Design review of the part built by this model. Coordinates are the model's own, in mm. A direction names the side the tool comes from. Give positions to 0.01 mm unless a question says otherwise; leave off trailing zeros. Loops run counter-clockwise (first coordinate to the right, second up) from the corner with the lowest first, then second, coordinate; pieces in that order, holes last. Notation, with made-up numbers: (83, -35) -> (121, -35) arc R21 ccw to (121, -15) -> close; hole circle Ø4 at (77.5, 30). An arc over 180 degrees is marked (long way). Use a Markdown table: item, result. Add a question column.
1. Add section C-C (z = 5.4). State the section outline as (x, y) points.
2. For faces 1 (the cylindrical face through (-10.46, -6.16, 4.04)), 2 (the flat face through (4.35, 2.465, 2.958)), 3 (the flat face through (7.5, 10, 3)), 4 (the flat face through (-4.556, -11.29, 2.958)), list the 3-axis set-ups (+Z, -Z, +X, -X, +Y, -Y) from which the entire face can be reached by the end or side of a thin tool; tool diameter is ignored.
3. To check wall thickness, follow line 1 (Z direction, x = -2, y = 12); line 2 (X direction, y = -8.25, z = 2.75); line 3 (X direction, y = -4.75, z = 4.1). State the ranges of each line that lie inside material, in increasing order.
4. Draft analysis for pull direction X (two halves, no side actions). For faces 5 (the flat face through (4.556, -11.29, 2.958)), 6 (the flat face through (0, 15, 3)), 7 (the cylindrical face through (9.58, -5.41, 3.32)), 8 (the flat face through (-7.5, 10, 3)), state which applies: pulls with the +X half, pulls with the -X half, needs draft (parallel to the pull), parting line crosses it, or undercut.
5. Add section D-D (z = 3). State the section outline as (x, y) points, and give its area (3 significant figures).
6. Add section A-A (y = 12). State the section outline as (x, z) points.
7. For pin 1 Ø2 at (y, z) = (8.5, 1.5) entering from -X; pin 2 Ø1.3 at (y, z) = (12, 3) entering from +X, all flat-tipped, find the tip position at first contact; note any pin that passes through.
8. Add section B-B (x = -5). State the section outline as (y, z) points.
```python
from build123d import *

# Parameters (mm, degrees)
F0_W     = 15
F0_H     = 15
F1_DEPTH = 6
F2_R     = 1.05
F3_DEPTH = 15
F5_COUNT = 3
F7_DEPTH = 6


with BuildPart() as f1:
    # F0 (on Top) → F1 (new body)
    with BuildSketch(Plane.XY):
        with Locations((0, 7.5)):
            Rectangle(F0_W, F0_H)
    extrude(amount=F1_DEPTH)

    # F2 (on face) → F3 (cut, through all)
    with BuildSketch(Plane(origin=(-7.5, 0, 0), x_dir=(0, -1, 0), z_dir=(-1, 0, 0))):
        with Locations((-12, 3)):
            Circle(F2_R)
    extrude(amount=-F3_DEPTH, mode=Mode.SUBTRACT)

    # F5: F1 ×3 about axis
    f5_axis = Axis((0, 0, -1.369192), (0, 0, -1))


with BuildPart() as f1_1:
    add(f1.part)
    for i in range(1, F5_COUNT):
        add(f1.part.rotate(f5_axis, i * 360 / F5_COUNT))

    # F6 (on Top) → F7 (cut, through all)
    with BuildSketch(Plane.XY):
        Polygon((2.886751, 5), (-2.886751, 5), (-5.773503, 0), (-2.886751, -5), (2.886751, -5), (5.773503, 0), align=None)
    extrude(amount=F7_DEPTH, mode=Mode.SUBTRACT)


solid = f1_1.part
```
Taken from the geometry:
| question | item | result |
|---|---|---|
| 1 | outline | (-16.74, -1) -> (-9.24, -14) -> (0, -8.66) -> (9.24, -14) -> (16.74, -1) -> (7.5, 4.33) -> (7.5, 15) -> (-7.5, 15) -> (-7.5, 4.33) -> close; hole (-5.77, 0) -> (-2.89, -5) -> (2.89, -5) -> (5.77, 0) -> (2.89, 5) -> (-2.89, 5) -> close |
| 2 | face 1 | none |
| 2 | face 2 | +Z, -Z |
| 2 | face 3 | +Z, -Z, +X, +Y |
| 2 | face 4 | +Z, -Z, -Y |
| 3 | line 1 | z = 0 to 1.95, 4.05 to 6 |
| 3 | line 2 | x = -12.56 to -10.27, -7.92 to 7.92, 10.27 to 12.56 |
| 3 | line 3 | x = -14.58 to -3.03, 3.03 to 14.58 |
| 4 | face 5 | undercut |
| 4 | face 6 | needs draft |
| 4 | face 7 | undercut |
| 4 | face 8 | pulls with the -X half |
| 5 | outline | (-16.74, -1) -> (-9.24, -14) -> (-7.55, -13.02) -> (-15.05, -0.03) -> close; (-13.23, 1.02) -> (-5.73, -11.97) -> (0, -8.66) -> (5.73, -11.97) -> (13.23, 1.02) -> (7.5, 4.33) -> (7.5, 10.95) -> (-7.5, 10.95) -> (-7.5, 4.33) -> close; (-7.5, 13.05) -> (7.5, 13.05) -> (7.5, 15) -> (-7.5, 15) -> close; (7.55, -13.02) -> (9.24, -14) -> (16.74, -1) -> (15.05, -0.03) -> close; hole (-5.77, 0) -> (-2.89, -5) -> (2.89, -5) -> (5.77, 0) -> (2.89, 5) -> (-2.89, 5) -> close |
| 5 | area | 396 mm^2 |
| 6 | outline | (-7.5, 0) -> (7.5, 0) -> (7.5, 1.95) -> (-7.5, 1.95) -> close; (-7.5, 4.05) -> (7.5, 4.05) -> (7.5, 6) -> (-7.5, 6) -> close |
| 7 | pin 1 | stops at x = -7.5 |
| 7 | pin 2 | passes through |
| 8 | outline | (-11.55, 0) -> (-1.34, 0) -> (-1.34, 6) -> (-11.55, 6) -> close; (1.34, 0) -> (15, 0) -> (15, 6) -> (1.34, 6) -> close; hole circle Ø2.1 at (12, 3) |
